```python
from build123d import *

# Parameters (mm, degrees)
SKETCH2_W                                       = 14.9
SKETCH2_H                                       = 11.3
SKETCH2_W_2                                     = 8.3
SKETCH2_H_2                                     = 7.3
BOSS_EXTRUDE1_DEPTH                             = 12.6
CUT_EXTRUDE1_DEPTH                              = 16.212659202
CUT_EXTRUDE1_DEPTH_BACK                         = 16.212659202
SKETCH4_W                                       = 4.6
SKETCH4_H                                       = 3.1
BOSS_EXTRUDE2_DEPTH                             = 3
CHAMFER1_SIZE                                   = 1
CHAMFER2_SIZE                                   = 0.8
CHAMFER3_SIZE                                   = 2
CSK_FOR_M3_FLAT_HEAD_MACHINE_SCREW1_D           = 3.6
CSK_FOR_M3_FLAT_HEAD_MACHINE_SCREW1_CSINK_D     = 6.3
CSK_FOR_M3_FLAT_HEAD_MACHINE_SCREW1_CSINK_ANGLE = 90
CHAMFER4_SIZE                                   = 2


with BuildPart() as part:
    # Sketch2 → Boss-Extrude1 (new body)
    with BuildSketch(Plane.XZ.offset(-12)):
        Rectangle(SKETCH2_W, SKETCH2_H)
        Rectangle(SKETCH2_W_2, SKETCH2_H_2, mode=Mode.SUBTRACT)
    extrude(amount=BOSS_EXTRUDE1_DEPTH)

    # Sketch4 → Cut-Extrude1 (cut, two sides: drawn at the far end of the back side and taken through both)
    with BuildSketch(Plane(origin=(0, 0, 0), x_dir=(0, 0, -1), z_dir=(1, 0, 0)).offset(-CUT_EXTRUDE1_DEPTH_BACK)):
        with Locations((0, 8.55)):
            Rectangle(SKETCH4_W, SKETCH4_H)
    extrude(amount=CUT_EXTRUDE1_DEPTH + CUT_EXTRUDE1_DEPTH_BACK, mode=Mode.SUBTRACT)

    # Sketch5 → Boss-Extrude2 (add)
    with BuildSketch(Plane.XZ.offset(0.6)):
        with BuildLine():
            Line((-20, 12.5), (20, 12.5))
            ThreePointArc((20, 12.5), (32.5, 0), (20, -12.5))
            Line((20, -12.5), (-20, -12.5))
            ThreePointArc((-20, -12.5), (-32.5, 0), (-20, 12.5))
        make_face()
    extrude(amount=BOSS_EXTRUDE2_DEPTH)

    # Chamfer1
    chamfer1_edges = [part.edges().sort_by_distance(p)[0] for p in [
        (-32.5, -3.6, 0),
        (0, -3.6, -12.5),
        (32.5, -3.6, 0),
        (0, -3.6, 12.5),
    ]]
    chamfer(chamfer1_edges, length=CHAMFER1_SIZE)

    # Chamfer2
    chamfer2_edges = [part.edges().sort_by_distance(p)[0] for p in [
        (0, 12, -3.65),
        (4.15, 12, 0),
        (0, 12, 3.65),
        (-4.15, 12, 0),
        (0, 12, -5.65),
        (-7.45, 12, 0),
        (0, 12, 5.65),
        (7.45, 12, 0),
    ]]
    chamfer(chamfer2_edges, length=CHAMFER2_SIZE)

    # Chamfer3
    # the kernel refuses this chamfer: 2 mm, written as the material it takes off along each edge
    with BuildSketch(Plane(origin=(-7.45, 16.343365976, 5.65), x_dir=(-0.027495876610586053, 0, -0.9996219169112968), z_dir=(0, -1, 0)), Plane(origin=(7.45, 16.343365976, 5.65), x_dir=(-0.9996219169112968, 0, 0.027495876610586487), z_dir=(0, -1, 0))) as chamfer3_piece_1:
        Polygon((CHAMFER3_SIZE * 0.999621916911, CHAMFER3_SIZE * 0.0274958766106), (-CHAMFER3_SIZE * 0.0274958766106, CHAMFER3_SIZE * 0.999621916911), (0, 0), align=None)
    extrude(amount=16.943365976, mode=Mode.SUBTRACT)
    with BuildSketch(Plane(origin=(-7.45, 16.343365976, -5.65), x_dir=(-0.027495876610586924, 0, 0.9996219169112968), z_dir=(0, -1, 0)), Plane(origin=(7.45, 16.343365976, -5.65), x_dir=(-0.9996219169112968, 0, -0.027495876610586487), z_dir=(0, -1, 0))) as chamfer3_piece_2:
        Polygon((CHAMFER3_SIZE * 0.999621916911, -CHAMFER3_SIZE * 0.0274958766106), (-CHAMFER3_SIZE * 0.0274958766106, -CHAMFER3_SIZE * 0.999621916911), (0, 0), align=None)
    extrude(amount=16.943365976, mode=Mode.SUBTRACT)

    # CSK for M3 Flat Head Machine Screw1 (through all)
    with Locations(Plane(origin=(0, -3.6, 0), x_dir=(-1, 0, 0), z_dir=(0, -1, 0))):
        with Locations((-20, 0), (19.948852039, 0)):
            CounterSinkHole(CSK_FOR_M3_FLAT_HEAD_MACHINE_SCREW1_D / 2, CSK_FOR_M3_FLAT_HEAD_MACHINE_SCREW1_CSINK_D / 2, counter_sink_angle=CSK_FOR_M3_FLAT_HEAD_MACHINE_SCREW1_CSINK_ANGLE)

    # Chamfer4
    chamfer4_edges = [part.edges().sort_by_distance(p)[0] for p in [
        (-7.45, -0.6, 0),
        (0, -0.6, 5.65),
        (0, -0.6, -5.65),
        (7.45, -0.6, 0),
        (-6.45, -0.6, 4.65),
        (-6.45, -0.6, -4.65),
        (6.45, -0.6, -4.65),
        (6.45, -0.6, 4.65),
    ]]
    chamfer(chamfer4_edges, length=CHAMFER4_SIZE)


solid = part.part
```
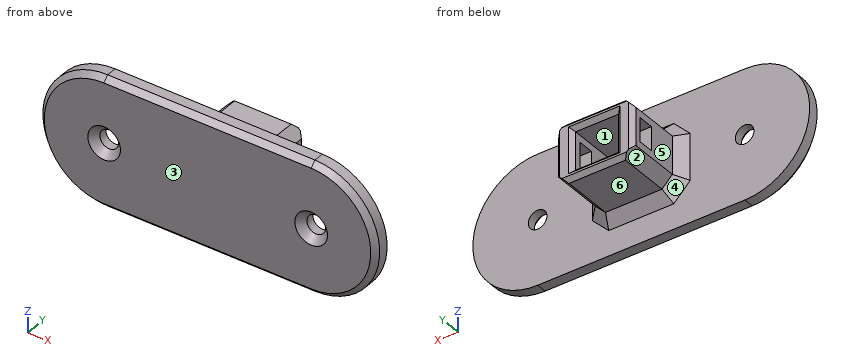
The listing builds one solid part. Answer for the finished solid, in the listing's coordinates (mm). Face numbers are marked on the shaded views. A direction names the side the tool comes from. Give positions to 0.01 mm unless a question says otherwise; leave off trailing zeros. Order: outer loops, then holes, each group sorted by start corner. A loop starts at its lowest first (then second) coordinate and runs counter-clockwise, first axis right, second up. Notation, with made-up numbers: M 26,-39 L 54,-39 A21 ccw 54,-17 Z; hole C -12.75,73.25 d2. An arc over 180 degrees is marked long. Put each result on its own line as item: value. Start each with the question number.
Item 1: The part is cut by section B-B, the plane x = -0.5. Determine the outline of the cut face in (y, z).
Item 2: The part is cut by section A-A, the plane y = 5.75. Determine the outline of the cut face in (x, z).
Item 3: Find the intervals of material crossed by line 1 along Z through (x, y) = (-3.5, 4.5); line 2 along Z through (x, y) = (20, -1.6); line 3 along X through (y, z) = (10.5, 0.25), in increasing order.
Item 4: For a pull along X with two mould halves and no side action, classify the marked faces 1, 2 and 3 as +X half, -X half, draft (parallel to the pull), parting line (faces both ways), or undercut.
Item 5: The part is cut by section D-D, the plane x = -13. Determine the outline of the cut face in (y, z).
Item 6: Which of the six approach directions +Z, -Z, +X, -X, +Y, -Y give full straight-line access (tool end or side, diameter ignored) to the marked faces 4, 5 and 6?
Item 7: Flat-ended cylindrical pins translate along their axes: P1, Ø3, axis at x = -0.5, y = 8.5, coming from the +Z side; P2, Ø6, axis at y = 4.5, z = 1, coming from the -X side; P3, Ø0.9, axis at x = -6.5, y = 8, coming from the -Z side. Find the tip coordinate at first contact, or state that the pin passes through.
Item 8: The part is cut by section C-C, the plane z = 0. State how many separate pieces and enclosed holes the cut face has, and give its area (3 significant figures).
Answer key:
1. outline: M -3.6,-11.5 L -2.6,-12.5 L -0.6,-12.5 L -0.6,-7.65 L 1.4,-5.65 L 11.2,-5.65 L 12,-4.85 L 12,-4.45 L 11.2,-3.65 L -0.6,-3.65 L -0.6,3.65 L 11.2,3.65 L 12,4.45 L 12,4.85 L 11.2,5.65 L 1.4,5.65 L -0.6,7.65 L -0.6,12.5 L -2.6,12.5 L -3.6,11.5 Z
2. outline: M -7.45,-3.65 L -5.45,-5.65 L 5.45,-5.65 L 7.45,-3.65 L 7.45,3.65 L 5.45,5.65 L -5.45,5.65 L -7.45,3.65 Z; hole M -4.15,-3.65 L 4.15,-3.65 L 4.15,3.65 L -4.15,3.65 Z
3. line 1: z = -5.65 to -3.65, 3.65 to 5.65
3. line 2: z = -12.5 to -1.8, 1.8 to 12.5
3. line 3: x = -7.45 to -4.15, 4.15 to 7.45
4. face 1: undercut
4. face 2: -X half
4. face 3: draft
5. outline: M -3.6,-11.5 L -2.6,-12.5 L -0.6,-12.5 L -0.6,12.5 L -2.6,12.5 L -3.6,11.5 Z
6. face 4: -Z, -X, +Y
6. face 5: +Z, -Z, -X, +Y
6. face 6: -Z, +X, -X, +Y
7. P1: stops at z = 5.65
7. P2: stops at x = -7.45
7. P3: stops at z = -5.05
8. separate pieces: 5
8. enclosed holes: 0
8. area: 234 mm²
